CAD build for the part. Positions are in the model's coordinates, mm. Face numbers are marked on the shaded views. A direction names the side the tool comes from. Coordinates: 2 decimals unless noted, no trailing zeros. Order: outer loops, then holes, each group sorted by start corner. A loop starts at its lowest first (then second) coordinate and runs counter-clockwise, first axis right, second up. Notation, with made-up numbers: M 29.25,35.25 L 87.25,35.25 A20 cw 87.25,53.25 Z; hole C 66,56.25 d8. An arc over 180 degrees is marked long. Write item = value, one per line. Start each with the question number.
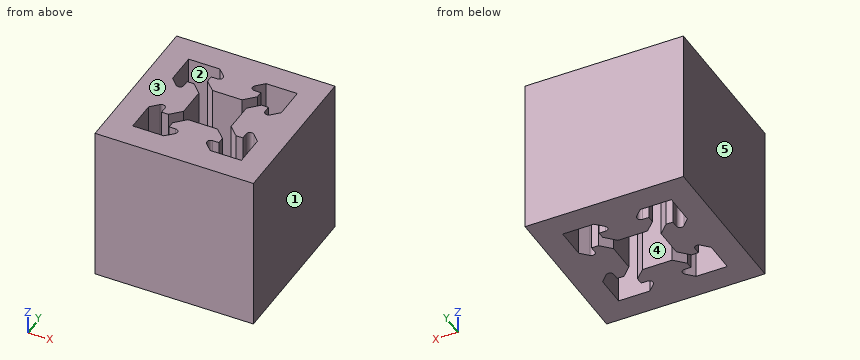
```python
from build123d import *

# Parameters (mm, degrees)
SKETCH1_W           = 30
SKETCH1_H           = 30
BOSS_EXTRUDE1_DEPTH = 30


with BuildPart() as part:
    # Sketch1 → Boss-Extrude1 (new body)
    with BuildSketch(Plane.XY):
        with Locations((15, 15)):
            Rectangle(SKETCH1_W, SKETCH1_H)
        with BuildLine():
            Line((17.802943725, 19.5), (12.197056275, 19.5))
            Line((12.197056275, 19.5), (10.289949494, 21.407106781))
            Line((10.289949494, 21.407106781), (10.289949494, 22.7))
            Line((10.289949494, 22.7), (11.517157288, 22.7))
            ThreePointArc((11.517157288, 22.7), (12.16387296, 23.132121597), (12.012132034, 23.894974747))
            Line((12.012132034, 23.894974747), (10.612132034, 25.294974747))
            Line((10.612132034, 25.294974747), (4.705025253, 25.294974747))
            Line((4.705025253, 25.294974747), (4.705025253, 19.387867966))
            Line((4.705025253, 19.387867966), (6.105025253, 17.987867966))
            ThreePointArc((6.105025253, 17.987867966), (6.867878403, 17.83612704), (7.3, 18.482842712))
            Line((7.3, 18.482842712), (7.3, 19.710050506))
            Line((7.3, 19.710050506), (8.592893219, 19.710050506))
            Line((8.592893219, 19.710050506), (10.5, 17.802943725))
            Line((10.5, 17.802943725), (10.5, 12.197056275))
            Line((10.5, 12.197056275), (8.592893219, 10.289949494))
            Line((8.592893219, 10.289949494), (7.3, 10.289949494))
            Line((7.3, 10.289949494), (7.3, 11.517157288))
            ThreePointArc((7.3, 11.517157288), (6.867878403, 12.16387296), (6.105025253, 12.012132034))
            Line((6.105025253, 12.012132034), (4.705025253, 10.612132034))
            Line((4.705025253, 10.612132034), (4.705025253, 4.705025253))
            Line((4.705025253, 4.705025253), (10.612132034, 4.705025253))
            Line((10.612132034, 4.705025253), (12.012132034, 6.105025253))
            ThreePointArc((12.012132034, 6.105025253), (12.16387296, 6.867878403), (11.517157288, 7.3))
            Line((11.517157288, 7.3), (10.289949494, 7.3))
            Line((10.289949494, 7.3), (10.289949494, 8.592893219))
            Line((10.289949494, 8.592893219), (12.197056275, 10.5))
            Line((12.197056275, 10.5), (17.802943725, 10.5))
            Line((17.802943725, 10.5), (19.710050506, 8.592893219))
            Line((19.710050506, 8.592893219), (19.710050506, 7.3))
            Line((19.710050506, 7.3), (18.482842712, 7.3))
            ThreePointArc((18.482842712, 7.3), (17.83612704, 6.867878403), (17.987867966, 6.105025253))
            Line((17.987867966, 6.105025253), (19.387867966, 4.705025253))
            Line((19.387867966, 4.705025253), (25.294974747, 4.705025253))
            Line((25.294974747, 4.705025253), (25.294974747, 10.612132034))
            Line((25.294974747, 10.612132034), (23.894974747, 12.012132034))
            ThreePointArc((23.894974747, 12.012132034), (23.132121597, 12.16387296), (22.7, 11.517157288))
            Line((22.7, 11.517157288), (22.7, 10.289949494))
            Line((22.7, 10.289949494), (21.407106781, 10.289949494))
            Line((21.407106781, 10.289949494), (19.5, 12.197056275))
            Line((19.5, 12.197056275), (19.5, 17.802943725))
            Line((19.5, 17.802943725), (21.407106781, 19.710050506))
            Line((21.407106781, 19.710050506), (22.7, 19.710050506))
            Line((22.7, 19.710050506), (22.7, 18.482842712))
            ThreePointArc((22.7, 18.482842712), (23.132121597, 17.83612704), (23.894974747, 17.987867966))
            Line((23.894974747, 17.987867966), (25.294974747, 19.387867966))
            Line((25.294974747, 19.387867966), (25.294974747, 25.294974747))
            Line((25.294974747, 25.294974747), (19.387867966, 25.294974747))
            Line((19.387867966, 25.294974747), (17.987867966, 23.894974747))
            ThreePointArc((17.987867966, 23.894974747), (17.83612704, 23.132121597), (18.482842712, 22.7))
            Line((18.482842712, 22.7), (19.710050506, 22.7))
            Line((19.710050506, 22.7), (19.710050506, 21.407106781))
            Line((19.710050506, 21.407106781), (17.802943725, 19.5))
        make_face(mode=Mode.SUBTRACT)
    extrude(amount=BOSS_EXTRUDE1_DEPTH)


solid = part.part
```
1. Mould opens along X. For the marked faces 3, 4 and 5 say: released by +X, released by -X, zero draft, split by the parting line, or undercut.
2. Slice it at B-B (x = 23.25). Write the cut outline in (y, z).
3. Slice it at A-A (y = 14.25). Write the cut outline in (x, z).
4. 3-axis set-ups, long thin cutter, end or side, ignore diameter. For the marked faces 1 and 2: which of +Z, -Z, +X, -X, +Y, -Y reach the whole face in a straight line?
5. Slice it at D-D (y = 20.5). Write the cut outline in (x, z).
6. Probe L1, parallel to X at y = 8, z = 27; L2, parallel to Y at x = 16.5, z = 10.75. List the from-to ranges inside material, lowest first.
Calculated:
q1.face_3 = zero draft
q1.face_4 = undercut
q1.face_5 = released by -X
q2.outline = M 0,0 L 4.71,0 L 4.71,30 L 0,30 Z; M 12.2,0 L 17.8,0 L 17.8,30 L 12.2,30 Z; M 25.29,0 L 30,0 L 30,30 L 25.29,30 Z
q3.outline = M 0,0 L 10.5,0 L 10.5,30 L 0,30 Z; M 19.5,0 L 30,0 L 30,30 L 19.5,30 Z
q4.face_1 = +Z, -Z, +X, +Y, -Y
q4.face_2 = +Z, -Z
q5.outline = M 0,0 L 4.71,0 L 4.71,30 L 0,30 Z; M 11.2,0 L 18.8,0 L 18.8,30 L 11.2,30 Z; M 25.29,0 L 30,0 L 30,30 L 25.29,30 Z
q6.L1 = 0 to 4.71, 10.29 to 19.71, 25.29 to 30
q6.L2 = 0 to 10.5, 19.5 to 30
